Work out the finished part from the listing and answer in its coordinate system (mm). Give positions to 0.01 mm unless a question says otherwise; leave off trailing zeros. Write each loop counter-clockwise with the first axis right and the second up, starting at its lowest first coordinate (ties: lowest second). Pieces come first, ordered by that corner, then holes.
1) Find section B-B (z = -47). Determine the outline of the cut face in (x, y), plus the area to 3 significant figures.
2) Straight lines are drawn through the part: probe 1 along Z at (x, y) = (40, 5.25); probe 2 along X at (y, z) = (2.25, -47); probe 3 along Z at (x, y) = (10, 4.5). For each, find the intervals that lie inside material, in ascending order.
3) Given pin 1 Ø2 at (x, y) = (98, 3.5) entering from +Z; pin 2 Ø8 at (x, z) = (10, -47) entering from +Y; pin 3 Ø3 at (x, y) = (10, 3.5) entering from +Z; pin 4 Ø1 at (y, z) = (2.5, 5.5) entering from +X, each flat-ended and moving along its own axis, determine where each tip first touches the part or whether it passes through.
4) Find section A-A (x = 10). Determine the outline of the cut face in (y, z), plus the area to 4 significant figures.
5) Find section C-C (y = 3.25). Determine the outline of the cut face in (x, z), plus the area to 3 significant figures.
6) Find section D-D (z = -23). Determine the outline of the cut face in (x, y), plus the area to 3 significant figures.
```python
from build123d import *

# Parameters (mm, degrees)
SKETCH_1_R      = 3
EXTRUDE_1_DEPTH = 6.5


with BuildPart() as part:
    # 스케치1 → 보스-돌출1 (new body)
    with BuildSketch(Plane(origin=(0, 0, 0), x_dir=(1, 0, 0), z_dir=(0, 1, 0))):
        with BuildLine():
            Line((0, 0), (0, 52))
            ThreePointArc((0, 52), (1.464466094, 55.535533906), (5, 57))
            Line((5, 57), (105, 57))
            ThreePointArc((105, 57), (108.535533906, 55.535533906), (110, 52))
            Line((110, 52), (110, 18))
            ThreePointArc((110, 18), (108.535533906, 14.464466094), (105, 13))
            Line((105, 13), (95, 13))
            ThreePointArc((95, 13), (91.464466094, 14.464466094), (90, 18))
            Line((90, 18), (90, 32))
            ThreePointArc((90, 32), (88.535533906, 35.535533906), (85, 37))
            Line((85, 37), (72.693946289, 37))
            ThreePointArc((72.693946289, 37), (70, 36.212202915), (68.154966925, 34.097061358))
            Line((68.154966925, 34.097061358), (49.077958727, -7.194122715))
            ThreePointArc((49.077958727, -7.194122715), (38.51023536, -12.888407421), (30.089287502, -4.333333333))
            ThreePointArc((30.089287502, -4.333333333), (28.425334196, -1.236136736), (25.133931253, 0))
            Line((25.133931253, 0), (0, 0))
        make_face()
        with Locations(Location((10, 47, 0), (0, 0, 90))):
            Circle(SKETCH_1_R, mode=Mode.SUBTRACT)
        with Locations(Location((40, -3, 0), (0, 0, 90))):
            Circle(SKETCH_1_R, mode=Mode.SUBTRACT)
        with Locations(Location((100, 23, 0), (0, 0, 90))):
            Circle(SKETCH_1_R, mode=Mode.SUBTRACT)
    extrude(amount=EXTRUDE_1_DEPTH)


solid = part.part
```
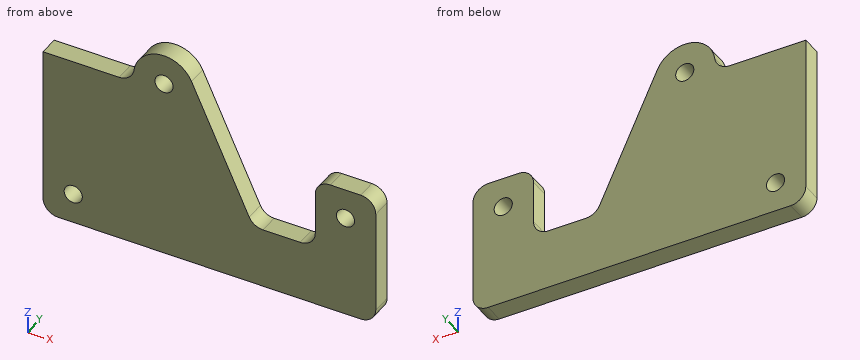
Results:
1. outline: (0, 0) - (7, 0) - (7, 6.5) - (0, 6.5) - close; (13, 0) - (110, 0) - (110, 6.5) - (13, 6.5) - close
1. area: 676 mm2
2. probe 1: z = -57 to 0, 6 to 13
2. probe 2: x = 0 to 7, 13 to 110
2. probe 3: z = -57 to -50, -44 to 0
3. pin 1: stops at z = -13
3. pin 2: stops at y = 6.5
3. pin 3: stops at z = 0
3. pin 4: stops at x = 50.09
4. outline: (0, -57) - (6.5, -57) - (6.5, -50) - (0, -50) - close; (0, -44) - (6.5, -44) - (6.5, 0) - (0, 0) - close
4. area: 331.5 mm2
5. outline: (0, -52) arc R5 ccw to (5, -57) - (105, -57) arc R5 ccw to (110, -52) - (110, -18) arc R5 ccw to (105, -13) - (95, -13) arc R5 ccw to (90, -18) - (90, -32) arc R5 cw to (85, -37) - (72.69, -37) arc R5 cw to (68.15, -34.1) - (49.08, 7.19) arc R10 ccw to (30.09, 4.33) arc R5 cw to (25.13, 0) - (0, 0) - close; hole circle Ø6 at (10, -47); hole circle Ø6 at (40, 3); hole circle Ø6 at (100, -23)
5. area: 5,060 mm2
6. outline: (0, 0) - (63.03, 0) - (63.03, 6.5) - (0, 6.5) - close; (90, 0) - (97, 0) - (97, 6.5) - (90, 6.5) - close; (103, 0) - (110, 0) - (110, 6.5) - (103, 6.5) - close
6. area: 501 mm2
